from build123d import *
from OCP.BRepFilletAPI import BRepFilletAPI_MakeChamfer

# Parameters (mm, degrees)
SKETCH1_W             = 24.646
SKETCH1_H             = 49.792
BOSS_EXTRUDE1_DEPTH   = 20
SKETCH2_W             = 27.686
SKETCH2_H             = 52.832
BOSS_EXTRUDE2_DEPTH   = 20
FILLET1_R             = 3.556
FILLET2_R             = 4.826
F_5_0MM_DOWEL_HOLE2_D = 5.4
CUT_EXTRUDE1_DEPTH    = 50.894225167
CUT_EXTRUDE2_START    = -4
CUT_EXTRUDE2_DEPTH    = 2
LPATTERN1_COUNT       = 4
LPATTERN1_PITCH       = 4
CHAMFER1_SIZE         = 2
CHAMFER1_SIZE2        = 1.154700538


with BuildPart() as part:
    # Sketch1 → Boss-Extrude1 (new body)
    with BuildSketch(Plane.XY):
        Rectangle(SKETCH1_W, SKETCH1_H)
    extrude(amount=BOSS_EXTRUDE1_DEPTH)

    # Sketch2 → Boss-Extrude2 (add)
    with BuildSketch(Plane.XY):
        Rectangle(SKETCH2_W, SKETCH2_H)
    extrude(amount=-BOSS_EXTRUDE2_DEPTH)

    # Fillet1
    fillet1_edges = [part.edges().sort_by_distance(p)[0] for p in [
        (-12.323, 24.896, 10),
        (12.323, 24.896, 10),
        (12.323, -24.896, 10),
        (-12.323, -24.896, 10),
    ]]
    fillet(fillet1_edges, radius=FILLET1_R)

    # Fillet2
    fillet2_edges = [part.edges().sort_by_distance(p)[0] for p in [
        (-13.843, -26.416, -10),
        (-13.843, 26.416, -10),
        (13.843, 26.416, -10),
        (13.843, -26.416, -10),
    ]]
    fillet(fillet2_edges, radius=FILLET2_R)

    # Ø5.0mm Dowel Hole2 (through all)
    with Locations(Plane(origin=(13.843, 0, 0), x_dir=(0, 0, -1), z_dir=(1, 0, 0))):
        with Locations((10, 16.256), (10, -16.256)):
            Hole(F_5_0MM_DOWEL_HOLE2_D / 2)

    # Sketch9 → Cut-Extrude1 (cut, through all)
    with BuildSketch(Plane.XY.offset(20)):
        with BuildLine():
            Line((7.243, -22.356), (-7.243, -22.356))
            ThreePointArc((-7.243, -22.356), (-9.039051224, -21.612051224), (-9.783, -19.816))
            Line((-9.783, -19.816), (-9.783, 19.816))
            ThreePointArc((-9.783, 19.816), (-9.039051224, 21.612051224), (-7.243, 22.356))
            Line((-7.243, 22.356), (7.243, 22.356))
            ThreePointArc((7.243, 22.356), (9.039051224, 21.612051224), (9.783, 19.816))
            Line((9.783, 19.816), (9.783, -19.816))
            ThreePointArc((9.783, -19.816), (9.039051224, -21.612051224), (7.243, -22.356))
        make_face()
    extrude(amount=-CUT_EXTRUDE1_DEPTH, mode=Mode.SUBTRACT)

    # Sketch10 → Cut-Extrude2 (cut)
    with BuildSketch(Plane.XY.offset(20).offset(CUT_EXTRUDE2_START)):
        with BuildLine():
            Line((-12.323, 21.34), (-12.323, -21.34))
            ThreePointArc((-12.323, -21.34), (-11.281471714, -23.854471714), (-8.767, -24.896))
            Line((-8.767, -24.896), (8.767, -24.896))
            ThreePointArc((8.767, -24.896), (11.281471714, -23.854471714), (12.323, -21.34))
            Line((12.323, -21.34), (12.323, 21.34))
            ThreePointArc((12.323, 21.34), (11.281471714, 23.854471714), (8.767, 24.896))
            Line((8.767, 24.896), (-8.767, 24.896))
            ThreePointArc((-8.767, 24.896), (-11.281471714, 23.854471714), (-12.323, 21.34))
        make_face()
        with BuildLine():
            Line((-11.823, 21.34), (-11.823, -21.34))
            ThreePointArc((-11.823, -21.34), (-10.927918323, -23.500918323), (-8.767, -24.396))
            Line((-8.767, -24.396), (8.767, -24.396))
            ThreePointArc((8.767, -24.396), (10.927918323, -23.500918323), (11.823, -21.34))
            Line((11.823, -21.34), (11.823, 21.34))
            ThreePointArc((11.823, 21.34), (10.927918323, 23.500918323), (8.767, 24.396))
            Line((8.767, 24.396), (-8.767, 24.396))
            ThreePointArc((-8.767, 24.396), (-10.927918323, 23.500918323), (-11.823, 21.34))
        make_face(mode=Mode.SUBTRACT)
    cut_extrude2 = extrude(amount=-CUT_EXTRUDE2_DEPTH, mode=Mode.SUBTRACT)

    # LPattern1: Cut-Extrude2 ×4
    with Locations(*[(0, 0, -i * LPATTERN1_PITCH) for i in range(1, LPATTERN1_COUNT)]):
        add(cut_extrude2, mode=Mode.SUBTRACT)

    # Chamfer1: one chamfer whose edges measure the first distance from different faces: ONE call of the kernel's chamfer builder (chamfer() names one face for all edges)
    chamfer1_edges_1 = [part.edges().sort_by_distance(p)[0] for p in [
        (0, -24.896, 20),
    ]]
    chamfer1_side_1 = [part.faces().sort_by_distance(p)[0] for p in [
        (0, -24.896, 18),
    ]]
    chamfer1_edges_2 = [part.edges().sort_by_distance(p)[0] for p in [
        (-12.323, 0, 20),
    ]]
    chamfer1_side_2 = [part.faces().sort_by_distance(p)[0] for p in [
        (-12.323, 0, 18),
    ]]
    chamfer1_edges_3 = [part.edges().sort_by_distance(p)[0] for p in [
        (12.323, 0, 20),
    ]]
    chamfer1_side_3 = [part.faces().sort_by_distance(p)[0] for p in [
        (12.323, 0, 18),
    ]]
    chamfer1_edges_4 = [part.edges().sort_by_distance(p)[0] for p in [
        (0, 24.896, 20),
    ]]
    chamfer1_side_4 = [part.faces().sort_by_distance(p)[0] for p in [
        (0, 24.896, 18),
    ]]
    chamfer1_edges_5 = [part.edges().sort_by_distance(p)[0] for p in [
        (-11.281471714, 23.854471714, 20),
    ]]
    chamfer1_side_5 = [part.faces().sort_by_distance(p)[0] for p in [
        (-11.281471714, 23.854471714, 18),
    ]]
    chamfer1_edges_6 = [part.edges().sort_by_distance(p)[0] for p in [
        (11.281471714, 23.854471714, 20),
    ]]
    chamfer1_side_6 = [part.faces().sort_by_distance(p)[0] for p in [
        (11.281471714, 23.854471714, 18),
    ]]
    chamfer1_edges_7 = [part.edges().sort_by_distance(p)[0] for p in [
        (11.281471714, -23.854471714, 20),
    ]]
    chamfer1_side_7 = [part.faces().sort_by_distance(p)[0] for p in [
        (11.281471714, -23.854471714, 18),
    ]]
    chamfer1_edges_8 = [part.edges().sort_by_distance(p)[0] for p in [
        (-11.281471714, -23.854471714, 20),
    ]]
    chamfer1_side_8 = [part.faces().sort_by_distance(p)[0] for p in [
        (-11.281471714, -23.854471714, 18),
    ]]
    chamfer1 = BRepFilletAPI_MakeChamfer(part.part.solid().wrapped)
    for e in chamfer1_edges_1:
        chamfer1.Add(CHAMFER1_SIZE, CHAMFER1_SIZE2, e.wrapped, chamfer1_side_1[0].wrapped)  # the first distance lies on this face
    for e in chamfer1_edges_2:
        chamfer1.Add(CHAMFER1_SIZE, CHAMFER1_SIZE2, e.wrapped, chamfer1_side_2[0].wrapped)  # the first distance lies on this face
    for e in chamfer1_edges_3:
        chamfer1.Add(CHAMFER1_SIZE, CHAMFER1_SIZE2, e.wrapped, chamfer1_side_3[0].wrapped)  # the first distance lies on this face
    for e in chamfer1_edges_4:
        chamfer1.Add(CHAMFER1_SIZE, CHAMFER1_SIZE2, e.wrapped, chamfer1_side_4[0].wrapped)  # the first distance lies on this face
    for e in chamfer1_edges_5:
        chamfer1.Add(CHAMFER1_SIZE, CHAMFER1_SIZE2, e.wrapped, chamfer1_side_5[0].wrapped)  # the first distance lies on this face
    for e in chamfer1_edges_6:
        chamfer1.Add(CHAMFER1_SIZE, CHAMFER1_SIZE2, e.wrapped, chamfer1_side_6[0].wrapped)  # the first distance lies on this face
    for e in chamfer1_edges_7:
        chamfer1.Add(CHAMFER1_SIZE, CHAMFER1_SIZE2, e.wrapped, chamfer1_side_7[0].wrapped)  # the first distance lies on this face
    for e in chamfer1_edges_8:
        chamfer1.Add(CHAMFER1_SIZE, CHAMFER1_SIZE2, e.wrapped, chamfer1_side_8[0].wrapped)  # the first distance lies on this face
    add(Compound.cast(chamfer1.Shape()), mode=Mode.REPLACE)


solid = part.part
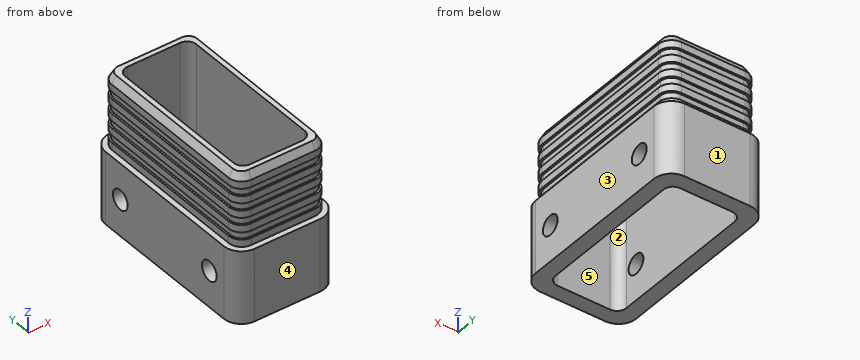
Design review of the part built by this model. Coordinates are the model's own, in mm. Face numbers are marked on the shaded views. A direction names the side the tool comes from. Round coordinates to 2 decimals unless told otherwise and drop trailing zeros. One line per item, written item: value. Start each with the question number.
Q1. Tool access review of the marked faces 4 and 5: name each direction out of +Z, -Z, +X, -X, +Y, -Y from which nothing blocks a thin tool from reaching the whole face with its end or side.
Q2. To check wall thickness, follow probe 1 along X at (y, z) = (19.5, -13); probe 2 along X at (y, z) = (18.5, 7); probe 3 along Y at (x, z) = (-12.15, -10). State the ranges of each line that lie inside material, in increasing order.
Q3. The part is to be moulded in two halves that separate along X. For the marked faces 1, 2 and 3, say which applies: pulls with the +X half, pulls with the -X half, needs draft (parallel to the pull), parting line crosses it, or undercut.
Q4. Add section A-A (z = -10). State how many separate pieces and enclosed holes the cut face has, then the cut area to 3 significant figures.
Q5. Insertion check: P1, Ø1.6, axis at x = 4, z = 3, coming from the +Y side; P2, Ø5, axis at y = 13.5, z = 5.5, coming from the +X side; P3, Ø6, axis at y = 16.256, z = -10, coming from the -X side; P4, Ø0.6, axis at x = -2.5, z = 10.5, coming from the -Y side. Each pin has a flat end and moves straight along its axis. Give the tip position at first contact, or say it passes through.
Response:
1. face 4: +Z, -Z, +X, -X, -Y
1. face 5: +Z, -Z
2. probe 1: x = -13.84 to -9.78, 9.78 to 13.84
2. probe 2: x = -11.82 to -9.78, 9.78 to 11.82
2. probe 3: y = -25.26 to -18.96, -13.56 to 13.56, 18.96 to 25.26
3. face 1: needs draft
3. face 2: undercut
3. face 3: pulls with the +X half
4. separate pieces: 4
4. enclosed holes: 0
4. area: 486 mm^2
5. P1: stops at y = 24.4
5. P2: stops at x = 12.32
5. P3: stops at x = -13.84
5. P4: stops at y = -24.4
